Source: three-view drawing plus pictorial views. Frame: mm from the lowest corner of the part. A direction names the side the tool comes from. Give positions to 0.01 mm unless a question says otherwise; leave off trailing zeros. Loops run counter-clockwise (first coordinate to the right, second up) from the corner with the lowest first, then second, coordinate; pieces in that order, holes last.
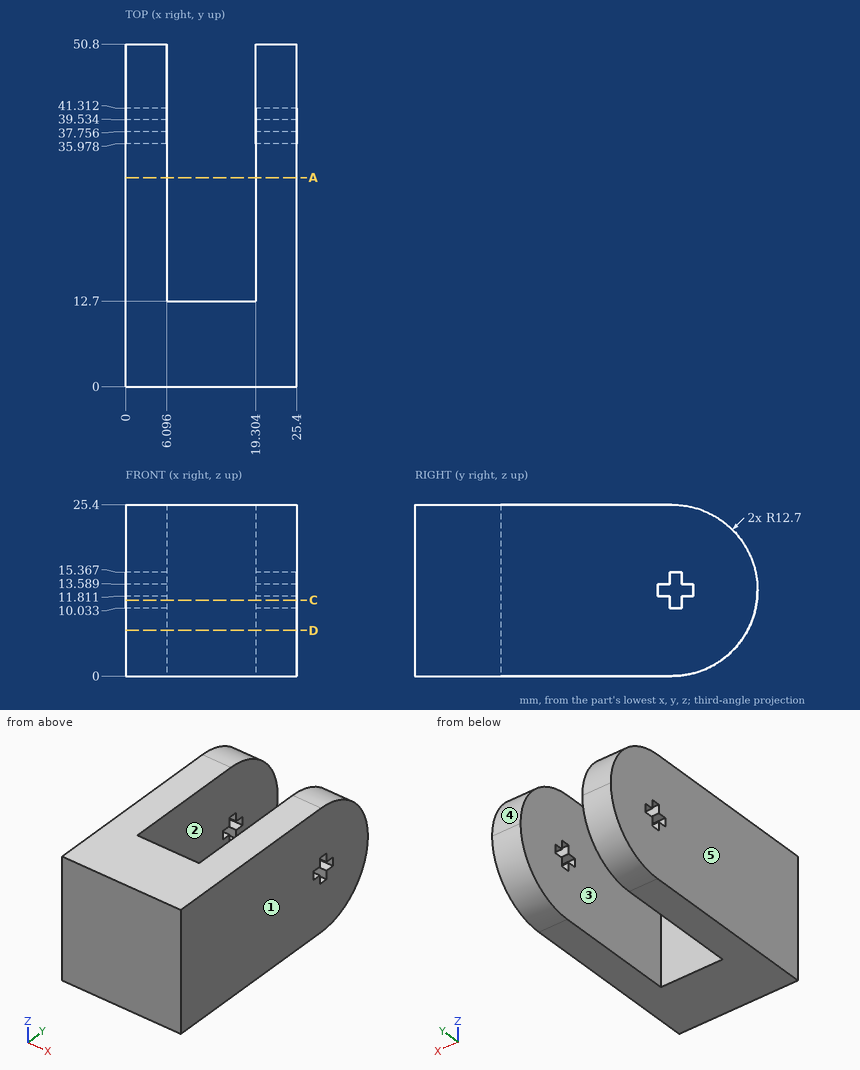
(1) Cut plane A-A (y = 31). Return the cut outline in (x, z).
Values follow:
outline: (0, 0) - (6.1, 0) - (6.1, 25.4) - (0, 25.4) - close; (19.3, 0) - (25.4, 0) - (25.4, 25.4) - (19.3, 25.4) - close
(2) Ray query, probe 1 along X at (y, z) = (36.5, 19.5); probe 2 along Y at (x, z) = (14.5, 20); probe 3 along Y at (x, z) = (4.5, 12). Return the intervals inside material, ascending.
Values follow:
probe 1: x = 0 to 6.1, 19.3 to 25.4
probe 2: y = 0 to 12.7
probe 3: y = 0 to 35.98, 41.31 to 50.78
(3) Cut plane C-C (z = 11.25). Return the cut outline in (x, y), and give its area (3 significant figures).
Values follow:
outline: (0, 0) - (25.4, 0) - (25.4, 37.76) - (19.3, 37.76) - (19.3, 12.7) - (6.1, 12.7) - (6.1, 37.76) - (0, 37.76) - close; (0, 39.53) - (6.1, 39.53) - (6.1, 50.72) - (0, 50.72) - close; (19.3, 39.53) - (25.4, 39.53) - (25.4, 50.72) - (19.3, 50.72) - close
area: 764 mm2
(4) Cut plane D-D (z = 6.75). Return the cut outline in (x, y).
Values follow:
outline: (0, 0) - (25.4, 0) - (25.4, 49.32) - (19.3, 49.32) - (19.3, 12.7) - (6.1, 12.7) - (6.1, 49.32) - (0, 49.32) - close
(5) Pin query (flat end, axial travel): pin 1 Ø1.4 at (x, y) = (3.5, 40.5) entering from -Z; pin 2 Ø2 at (x, z) = (3, 11) entering from +Y; pin 3 Ø6 at (x, z) = (13, 9) entering from +Y; pin 4 Ø6 at (x, y) = (11, 41) entering from +Z. Return the tip coordinate at first contact, or that it passes through.
Values follow:
pin 1: stops at z = 0.11
pin 2: stops at y = 50.78
pin 3: stops at y = 12.7
pin 4: passes through
(6) Reachability of the marked faces 1 and 2 from +Z, -Z, +X, -X, +Y, -Y: full face, straight path, thin tool, end or side. Return the list, or none.
Values follow:
face 1: +Z, -Z, +X, +Y, -Y
face 2: +Z, -Z, +Y
(7) Mould query, pull axis X, two halves, no side actions, for the marked faces 3, 4 and 5. Classes: +X half, -X half, draft (parallel to the pull), parting line (faces both ways), or undercut.
Values follow:
face 3: undercut
face 4: draft
face 5: -X half
